from build123d import *

# Parameters (mm, degrees)
BOSS_EXTRUDE1_DEPTH = 10
SKETCH2_W           = 80
SKETCH2_H           = 10
BOSS_EXTRUDE2_DEPTH = 20


with BuildPart() as part:
    # Sketch1 → Boss-Extrude1 (new body)
    with BuildSketch(Plane(origin=(0, 0, 0), x_dir=(0, 0, -1), z_dir=(1, 0, 0))):
        Polygon((0, 0), (80, 0), (80, 74.5), (66.25, 74.5), (66.25, 69.5), (70.25, 69.5), (70.25, 62.1), (9.75, 62.1), (9.75, 69.5), (13.75, 69.5), (13.75, 74.5), (0, 74.5), align=None)
    extrude(amount=BOSS_EXTRUDE1_DEPTH)

    # Sketch2 → Boss-Extrude2 (add)
    with BuildSketch(Plane(origin=(10, 0, 0), x_dir=(0, 0, -1), z_dir=(1, 0, 0))):
        with Locations((40, 5)):
            Rectangle(SKETCH2_W, SKETCH2_H)
    extrude(amount=BOSS_EXTRUDE2_DEPTH)


solid = part.part
Model file for the job. Use its own axes, mm. A direction names the side the tool comes from. Coordinates: 2 decimals unless noted, no trailing zeros. Loops run counter-clockwise (first coordinate to the right, second up) from the corner with the lowest first, then second, coordinate; pieces in that order, holes last. Notation, with made-up numbers: (85.25, 79.5) -> (117.25, 79.5) arc R13 cw to (117.25, 94.5) -> close; hole circle Ø10 at (-12, 15). An arc over 180 degrees is marked (long way). Use one line per item in the form item = value. Start each with the question number.
(1) Probe probe 1 along Y at (x, z) = (7.75, -69); probe 2 along Y at (x, z) = (22.5, -62). List the from-to ranges inside material, lowest first. Write a range as from..to.
(2) Cut at C-C on y = 42. Give the cut face in (x, z), and give its area (3 significant figures).
(3) Cut at B-B on z = -17. Give the cut face in (x, y).
(4) Pull direction Z, two halves, no side cores. Call faces 4 (the flat face through (5, 72, -66.25)), 5 (the flat face through (0, 29, -39)), 6 (the flat face through (8, 28, 0)): pulls with the +Z half, pulls with the -Z half, needs draft (parallel to the pull), parting line crosses it, or undercut.
(5) Cut at A-A on x = 8. Give the cut face in (y, z).
(6) Flat gauge pins, fed straight in: pin 1 (16 mm diameter, centred on x = 16, z = -52, fed in from +Y); pin 2 (19.5 mm diameter, centred on y = 40, z = -22.5, fed in from +X). Where does each tip first touch, or does it go through?
(7) Tool access for faces 1 (the flat face through (5, 72, -13.75)), 2 (the flat face through (5, 66, -9.75)), 3 (the flat face through (20, 10, -39)): list every direction of +Z, -Z, +X, -X, +Y, -Y with a clear straight run to the whole face (end or side of a thin tool).
(8) Cut at D-D on z = -73. Give the cut face in (x, y).
Values:
q1.probe_1 = 0..62.1, 69.5..74.5
q1.probe_2 = 0..10
q2.outline = (0, -80) -> (10, -80) -> (10, 0) -> (0, 0) -> close
q2.area = 800 mm2
q3.outline = (0, 0) -> (30, 0) -> (30, 10) -> (10, 10) -> (10, 62.1) -> (0, 62.1) -> close
q4.face_4 = undercut
q4.face_5 = needs draft
q4.face_6 = pulls with the +Z half
q5.outline = (0, -80) -> (74.5, -80) -> (74.5, -66.25) -> (69.5, -66.25) -> (69.5, -70.25) -> (62.1, -70.25) -> (62.1, -9.75) -> (69.5, -9.75) -> (69.5, -13.75) -> (74.5, -13.75) -> (74.5, 0) -> (0, 0) -> close
q6.pin_1 = 62.1
q6.pin_2 = 10
q7.face_1 = +X, -X, +Y
q7.face_2 = +X, -X
q7.face_3 = +Z, -Z, +X, +Y
q8.outline = (0, 0) -> (30, 0) -> (30, 10) -> (10, 10) -> (10, 74.5) -> (0, 74.5) -> close
